from build123d import *

# Parameters (mm, degrees)
F1_DEPTH = 25
F3_W     = 25
F3_H     = 4.25
F4_DEPTH = 55
F5_W     = 25
F5_H     = 5
F6_DEPTH = 7
F7_R     = 5
F8_R     = 5


# Not quite as in the source:
# - a feature of the source that left no trace in its solid (it failed there, or was rolled back) is left out


with BuildPart() as f1:
    # F0 (on Right) → F1 (new body)
    with BuildSketch(Plane.YZ):
        Polygon((17.6, 0.1), (17.6, -10.15), (16.6, -10.15), (16.6, -14.15), (21.6, -14.15), (21.6, 4.1), (0, 4.1), (-21.6, 4.1), (-21.6, -14.15), (-16.6, -14.15), (-16.6, -10.15), (-17.6, -10.15), (-17.6, 0.1), (0, 0.1), align=None)
    extrude(amount=F1_DEPTH)

    # F3 (on face) → F4 (join)
    with BuildSketch(Plane.XZ.offset(21.6)):
        with Locations((12.5, -5.025)):
            Rectangle(F3_W, F3_H)
    extrude(amount=F4_DEPTH)

    # F5 (on face) → F6 (join, through all)
    with BuildSketch(Plane.XY.offset(-2.9)):
        with Locations((12.5, -74.1)):
            Rectangle(F5_W, F5_H)
    extrude(amount=F6_DEPTH)

    # F7
    f7_edges = [f1.edges().sort_by_distance(p)[0] for p in [
        (12.5, -21.6, -2.9),
        (12.5, -21.6, -7.15),
        (12.5, -71.6, -2.9),
        (12.5, -76.6, -7.15),
    ]]
    fillet(f7_edges, radius=F7_R)

    # F8
    f8_edges = [f1.edges().sort_by_distance(p)[0] for p in [
        (0, -74.1, 4.1),
        (25, -74.1, 4.1),
    ]]
    fillet(f8_edges, radius=F8_R)


solid = f1.part
For this review, take the finished solid that the model builds, in its own axes (mm). A direction names the side the tool comes from. Round coordinates to 2 decimals unless told otherwise and drop trailing zeros. Loops run counter-clockwise (first coordinate to the right, second up) from the corner with the lowest first, then second, coordinate; pieces in that order, holes last. Notation, with made-up numbers: (28.5, 27) - (33.5, 27) arc R16 cw to (33.5, 56) - close; hole circle Ø10 at (32.5, -12.5). An arc over 180 degrees is marked (long way). Answer as CSV lines item,"result".
(1) Consider section D-D on z = -8. Give the boundary of the cut face in (x, y), then the cut area to 3 significant figures.
Checked values:
outline,"(0, -23.81) - (25, -23.81) - (25, -17.6) - (0, -17.6) - close; (0, 17.6) - (25, 17.6) - (25, 21.6) - (0, 21.6) - close"
area,"255 mm2"
(2) Consider section A-A on z = 1. Give the boundary of the cut face in (x, y), then the cut area to 3 significant figures.
Checked values:
outline,"(0, -21.72) - (25, -21.72) - (25, 21.6) - (0, 21.6) - close; (0.38, -76.6) - (24.62, -76.6) - (24.62, -71.48) - (0.38, -71.48) - close"
area,"1,210 mm2"
(3) Consider section B-B on x = 17.25. Give the boundary of the cut face in (y, z), then the cut area to 3 significant figures.
Checked values:
outline,"(-76.6, -2.15) arc R5 ccw to (-71.6, -7.15) - (-26.6, -7.15) arc R5 cw to (-21.6, -12.15) - (-21.6, -14.15) - (-16.6, -14.15) - (-16.6, -10.15) - (-17.6, -10.15) - (-17.6, 0.1) - (17.6, 0.1) - (17.6, -10.15) - (16.6, -10.15) - (16.6, -14.15) - (21.6, -14.15) - (21.6, 4.1) - (-21.6, 4.1) - (-21.6, 2.1) arc R5 cw to (-26.6, -2.9) - (-66.6, -2.9) arc R5 cw to (-71.6, 2.1) - (-71.6, 4.1) - (-76.6, 4.1) - close"
area,"574 mm2"
(4) Insertion check: P1, Ø4.5, axis at x = 8, z = -13, coming from the -Y side; P2, Ø10, axis at x = 6, z = -5, coming from the -Y side; P3, Ø2, axis at x = 15, z = -13, coming from the -Y side; P4, Ø12.5, axis at x = 13, y = -51.5, coming from the +Z side. Each pin has a flat end and moves straight along its axis. Give the tip position at first contact, or say it passes through.
Checked values:
P1,"stops at y = -21.8"
P2,"stops at y = -76.6"
P3,"stops at y = -21.6"
P4,"stops at z = -2.9"
(5) Tool access review of faces 1 (the face through (12.68, -70.1, -1.47)), 2 (the face through (23.5, -74.22, 2.67)), 3 (the face through (12, 17.6, -5)), 4 (the face through (1.43, -74.22, 2.6)), 5 (the face through (12, -49, -7.15)): name each direction out of +Z, -Z, +X, -X, +Y, -Y from which nothing blocks a thin tool from reaching the whole face with its end or side.
Checked values:
face 1,"+Z, +X, -X"
face 2,"+Z, +X, -Y"
face 3,"+X, -X"
face 4,"+Z, -X, -Y"
face 5,"-Z, +X, -X, -Y"
(6) Consider section C-C on y = -64. Give the boundary of the cut face in (x, z).
Checked values:
outline,"(0, -7.15) - (25, -7.15) - (25, -2.9) - (0, -2.9) - close"
(7) Wall thickness on line 1 (Y direction, x = 15.25, z = 2.25); line 2 (Y direction, x = 5, z = -11.75); line 3 (Z direction, x = 15, y = -9.5): over which ranges is each line inside the solid? List them lowest first.
Checked values:
line 1,"y = -76.6 to -71.6, -21.6 to 21.6"
line 2,"y = -21.62 to -16.6, 16.6 to 21.6"
line 3,"z = 0.1 to 4.1"
(8) Mouldability with a two-part tool opening along Y and no side actions: class faces 6 (the face through (12, 21.6, -5)), 7 (the face through (12, -21.6, -13)), 8 (the face through (12, -21.6, 3)) as +Y half, -Y half, draft (parallel to the pull), parting line (faces both ways), or undercut.
Checked values:
face 6,"+Y half"
face 7,"-Y half"
face 8,"undercut"
